from build123d import *

# Parameters (mm, degrees)
SKETCH_1_W          = 20
SKETCH_1_H          = 10
SKETCH_1_R          = 1
EXTRUDE_1_DEPTH     = 5
SKETCH_2_R          = 1
EXTRUDE_2_DEPTH     = 2.5
SKETCH_4_R          = 2
CUT_EXTRUDE_2_DEPTH = 3


with BuildPart() as part:
    # 草图1 → 凸台-拉伸1 (new body)
    with BuildSketch(Plane.XY):
        Rectangle(SKETCH_1_W, SKETCH_1_H)
        with Locations((-5, 0)):
            Circle(SKETCH_1_R, mode=Mode.SUBTRACT)
        with Locations((5, 0)):
            Circle(SKETCH_1_R, mode=Mode.SUBTRACT)
    extrude(amount=EXTRUDE_1_DEPTH)

    # 草图2 → 凸台-拉伸2 (add)
    with BuildSketch(Plane.XY.offset(5)):
        Circle(SKETCH_2_R)
    extrude(amount=EXTRUDE_2_DEPTH)

    # 草图4 → 切除-拉伸2 (cut)
    with BuildSketch(Plane.XY.offset(5)):
        with Locations((5, 0)):
            Circle(SKETCH_4_R)
        with Locations((-5, 0)):
            Circle(SKETCH_4_R)
    extrude(amount=-CUT_EXTRUDE_2_DEPTH, mode=Mode.SUBTRACT)


solid = part.part
Here's how the part is built. I have some questions about the finished solid (model axes, mm). A direction names the side the tool comes from. Coordinates: 2 decimals unless noted, no trailing zeros. Loops run counter-clockwise (first coordinate to the right, second up) from the corner with the lowest first, then second, coordinate; pieces in that order, holes last. Notation, with made-up numbers: (5.5, 75) -> (45.5, 75) arc R33 cw to (45.5, 103) -> close; hole circle Ø8 at (72, 10). An arc over 180 degrees is marked (long way). Use one line per item in the form item = value. Start each with the question number.
(1) We'd pull the mould along X, two halves only. Please class faces 3 (the face through (4.2, -0.6, 1)), 4 (the face through (0, 0, 7.5)), 5 (the face through (-5.8, -0.6, 1)), 6 (the face through (10, 0, 2)): pulls with the +X half, pulls with the -X half, needs draft (parallel to the pull), parting line crosses it, or undercut.
(2) If we section it at A-A (x = -5): Please give me the cut outline in (y, z), then the cut area to 3 significant figures.
(3) Will these pins go through, and if not, where does the flat tip stop? pin 1 (1.2 mm diameter, centred on x = 5, y = 0, fed in from -Z); pin 2 (2 mm diameter, centred on x = -5.5, y = 4, fed in from +Z); pin 3 (1.2 mm diameter, centred on x = 5.5, y = 1, fed in from +Z).
(4) If we section it at B-B (y = 0): Please give me the cut outline in (x, z), then the cut area to 3 significant figures.
(5) Please list where these lines run through material, in increasing order: line 1 along X through (y, z) = (0, 0.75); line 2 along Y through (x, z) = (5, 0.6); line 3 along Y through (x, z) = (-5, 3.25).
(6) On a 3-axis mill with a long thin cutter (end or side, diameter ignored), from which of +Z, -Z, +X, -X, +Y, -Y can I reach the whole of each face in a straight line? I mean faces 1 (the face through (-10, 0, 2)), 2 (the face through (-4, -1, 2)). Say none if no direction works.
(7) If we section it at C-C (z = 4.75): Please give me the cut outline in (x, y).
(8) If we section it at D-D (x = 0): Please give me the cut outline in (y, z).
Verdict:
q1.face_3 = undercut
q1.face_4 = needs draft
q1.face_5 = undercut
q1.face_6 = pulls with the +X half
q2.outline = (-5, 0) -> (-1, 0) -> (-1, 2) -> (-2, 2) -> (-2, 5) -> (-5, 5) -> close; (1, 0) -> (5, 0) -> (5, 5) -> (2, 5) -> (2, 2) -> (1, 2) -> close
q2.area = 34.0 mm²
q3.pin_1 = through
q3.pin_2 = 5
q3.pin_3 = 2
q4.outline = (-10, 0) -> (-6, 0) -> (-6, 2) -> (-7, 2) -> (-7, 5) -> (-10, 5) -> close; (-4, 0) -> (4, 0) -> (4, 2) -> (3, 2) -> (3, 5) -> (1, 5) -> (1, 7.5) -> (-1, 7.5) -> (-1, 5) -> (-3, 5) -> (-3, 2) -> (-4, 2) -> close; (6, 0) -> (10, 0) -> (10, 5) -> (7, 5) -> (7, 2) -> (6, 2) -> close
q4.area = 73.0 mm²
q5.line_1 = -10 to -6, -4 to 4, 6 to 10
q5.line_2 = -5 to -1, 1 to 5
q5.line_3 = -5 to -2, 2 to 5
q6.face_1 = +Z, -Z, -X, +Y, -Y
q6.face_2 = +Z
q7.outline = (-10, -5) -> (10, -5) -> (10, 5) -> (-10, 5) -> close; hole circle Ø4 at (-5, 0); hole circle Ø4 at (5, 0)
q8.outline = (-5, 0) -> (5, 0) -> (5, 5) -> (1, 5) -> (1, 7.5) -> (-1, 7.5) -> (-1, 5) -> (-5, 5) -> close
